Geometry: final body of the model. Coordinates: model frame, mm. A direction names the side the tool comes from. Give positions to 0.01 mm unless a question says otherwise; leave off trailing zeros. Write each loop counter-clockwise with the first axis right and the second up, starting at its lowest first coordinate (ties: lowest second). Pieces come first, ordered by that corner, then holes.
Q1. Cut plane B-B on y = -1. Return the cut outline in (x, z).
Q2. Pin query (flat end, axial travel): pin 1 (2 mm diameter, centred on x = -3.5, y = -4.5, fed in from +Z); pin 2 (1.1 mm diameter, centred on x = 0, z = 3.5, fed in from -Y) (3 decimals); pin 3 (1.5 mm diameter, centred on x = 0.5, z = 3, fed in from +Y). Return the tip coordinate at first contact, or that it passes through.
Q3. Draft query along Y for faces 1 (the face through (0, 2, 2.5)), 2 (the face through (7.5, 0, 1)), 3 (the face through (0, -10, 1)). Return one class per face: pulls with the +Y half, pulls with the -Y half, needs draft (parallel to the pull), parting line crosses it, or undercut.
Q4. Cut plane C-C on x = 5.75. Return the cut outline in (y, z), plus the area to 3 significant figures.
Q5. Cut plane A-A on z = 3.4. Return the cut outline in (x, y) (3 decimals).
Q6. Line query: L1, parallel to Z at x = 3.75, y = 0.25; L2, parallel to X at y = 2.5, z = 2.35; L3, parallel to Z at x = 1.5, y = -3.5. Output: solid intervals per line, ascending.
Q7. Cut plane D-D on y = -6.75. Return the cut outline in (x, z), plus the area to 3 significant figures.
Q8. Reachability of faces 4 (the face through (-2, 0, 3)), 5 (the face through (0, -2, 2.5)), 6 (the face through (0, 3.225, 3)), 7 (the face through (7.215, 9.699, 1.014)) from +Z, -Z, +X, -X, +Y, -Y: full face, straight path, thin tool, end or side. Return the list, or none.
```python
from build123d import *

# Parameters (mm, degrees)
F0_W     = 15
F0_H     = 20
F1_DEPTH = 2
F0_W_2   = 4
F0_H_2   = 0.775
F0_H_3   = 1.05
F2_DEPTH = 2.5
F0_H_4   = 0.45
F3_DEPTH = 4
F4_SIZE  = 0.1
F5_R     = 1


with BuildPart() as f1:
    # F0 (on Top) → F1 (new body)
    with BuildSketch(Plane.XY):
        Rectangle(F0_W, F0_H)
        Polygon((2, -3.225), (2, -4), (-2, -4), (-2, -3.225), (-2, -2.775), (-2, -1.725), (-2, -1.275), (-2, -0.225), (-2, 0), (-2, 0.107463), (-2, 0.225), (-2, 1.275), (-2, 1.725), (-2, 2.775), (-2, 3.225), (-2, 4), (2, 4), (2, 3.225), (2, 2.775), (2, 1.725), (2, 1.275), (2, 0.225), (2, -0.225), (2, -1.275), (2, -1.725), (2, -2.775), align=None, mode=Mode.SUBTRACT)
    extrude(amount=F1_DEPTH)

    # F0 (on Top) → F2 (join)
    with BuildSketch(Plane.XY):
        with Locations((0, 3.6125)):
            Rectangle(F0_W_2, F0_H_2)
        with Locations((0, 0.75)):
            Rectangle(F0_W_2, F0_H_3)
        with Locations((0, -0.75)):
            Rectangle(F0_W_2, F0_H_3)
        with Locations((0, -3.6125)):
            Rectangle(F0_W_2, F0_H_2)
        with Locations((0, 2.25)):
            Rectangle(F0_W_2, F0_H_3)
        with Locations((0, -2.25)):
            Rectangle(F0_W_2, F0_H_3)
    extrude(amount=F2_DEPTH)

    # F0 (on Top) → F3 (join)
    with BuildSketch(Plane.XY):
        with Locations((0, 1.5)):
            Rectangle(F0_W_2, F0_H_4)
        Polygon((-2, -0.225), (2, -0.225), (2, 0.225), (-2, 0.225), (-2, 0.107463), (-2, 0), align=None)
        with Locations((0, -1.5)):
            Rectangle(F0_W_2, F0_H_4)
        with Locations((0, 3)):
            Rectangle(F0_W_2, F0_H_4)
        with Locations((0, -3)):
            Rectangle(F0_W_2, F0_H_4)
    extrude(amount=F3_DEPTH)

    # F4
    f4_edges = [f1.edges().sort_by_distance(p)[0] for p in [
        (0, -1.725, 4),
        (0, -1.275, 4),
        (0, -0.225, 4),
        (0, 0.225, 4),
        (0, 1.275, 4),
        (0, 1.725, 4),
        (0, 2.775, 4),
        (0, 3.225, 4),
        (0, -3.225, 4),
        (0, -2.775, 4),
    ]]
    chamfer(f4_edges, length=F4_SIZE)

    # F5
    f5_edges = [f1.edges().sort_by_distance(p)[0] for p in [
        (7.5, 10, 1),
        (7.5, -10, 1),
        (-7.5, -10, 1),
        (-7.5, 10, 1),
    ]]
    fillet(f5_edges, radius=F5_R)


solid = f1.part
```
Data:
1. outline: (-7.5, 0) - (7.5, 0) - (7.5, 2) - (2, 2) - (2, 2.5) - (-2, 2.5) - (-2, 2) - (-7.5, 2) - close
2. pin 1: stops at z = 2
2. pin 2: stops at y = -3.225
2. pin 3: stops at y = 4
3. face 1: undercut
3. face 2: needs draft
3. face 3: pulls with the -Y half
4. outline: (-10, 0) - (10, 0) - (10, 2) - (-10, 2) - close
4. area: 40.0 mm2
5. outline: (-2, -3.225) - (2, -3.225) - (2, -2.775) - (-2, -2.775) - close; (-2, -1.725) - (2, -1.725) - (2, -1.275) - (-2, -1.275) - close; (-2, -0.225) - (2, -0.225) - (2, 0.225) - (-2, 0.225) - close; (-2, 1.275) - (2, 1.275) - (2, 1.725) - (-2, 1.725) - close; (-2, 2.775) - (2, 2.775) - (2, 3.225) - (-2, 3.225) - close
6. L1: z = 0 to 2
6. L2: x = -2 to 2
6. L3: z = 0 to 2.5
7. outline: (-7.5, 0) - (7.5, 0) - (7.5, 2) - (-7.5, 2) - close
7. area: 30.0 mm2
8. face 4: +Z, -X, +Y, -Y
8. face 5: +Z, +X, -X
8. face 6: +Z, +X, -X, +Y
8. face 7: +Z, -Z, +X, +Y
